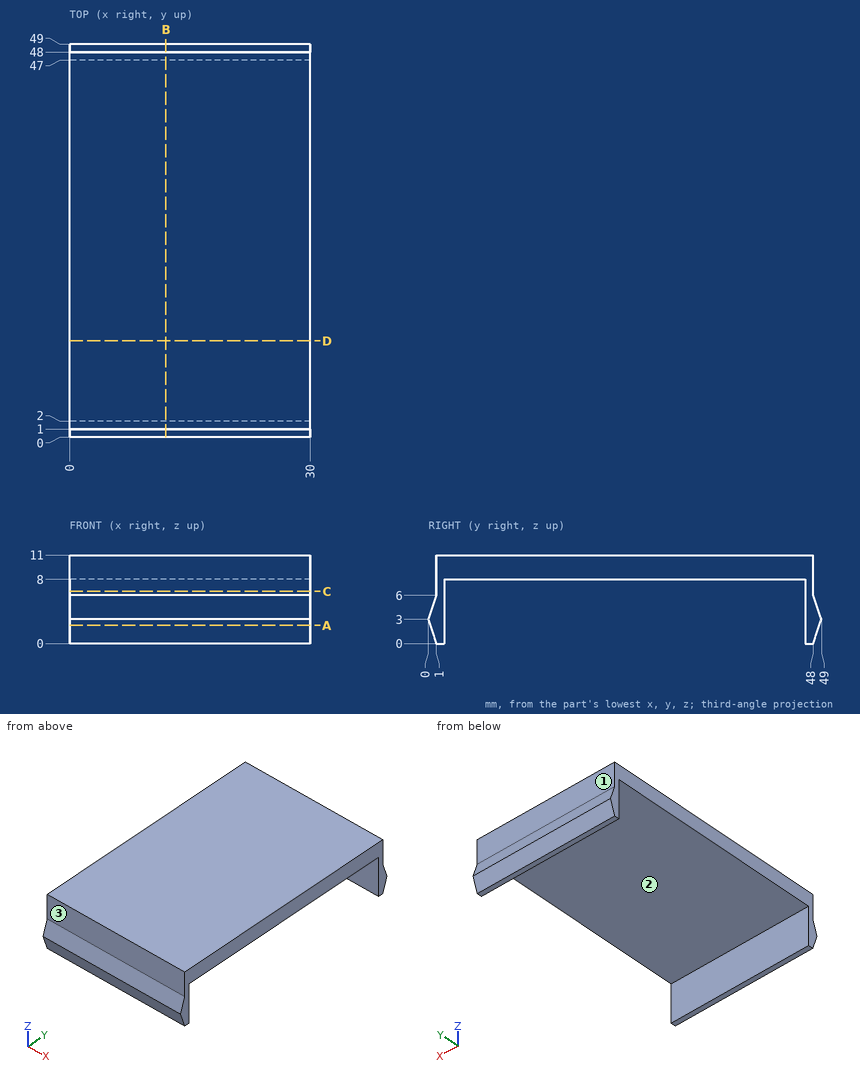
Design review of the part shown in the three views and the two pictorial views. Dimensions are in mm from the part's minimum x, y and z. A direction names the side the tool comes from. Round coordinates to 2 decimals unless told otherwise and drop trailing zeros. Loops run counter-clockwise (first coordinate to the right, second up) from the corner with the lowest first, then second, coordinate; pieces in that order, holes last. Notation, with made-up numbers: (-33.5, -20.75) -> (-17.5, -20.75) arc R18 ccw to (-17.5, 6.25) -> close; hole circle Ø1 at (42, -9). An arc over 180 degrees is marked (long way). Use one line per item in the form item = value. Start each with the question number.
Q1. Machinability: for the marked faces 1, 2 and 3, which of the approach directions +Z, -Z, +X, -X, +Y, -Y give a long, thin tool a straight path to every point of the face, cutting with its end or side? Answer none if there is none.
Q2. We need section B-B on x = 12. Give the boundary of the cut face in (y, z).
Q3. We need section C-C on z = 6.5. Give the boundary of the cut face in (x, y), then the cut area to 3 significant figures.
Q4. Wall thickness on line 1 along Y through (x, z) = (8.75, 7); line 2 along Y through (x, z) = (16, 4.5); line 3 along Z through (x, y) = (28, 32): over which ranges is each line inside the solid? List them lowest first. Write a range as [from, to].
Q5. For pin 1 Ø4 at (x, z) = (21.5, 9.5) entering from +Y; pin 2 Ø4 at (x, z) = (19, 9.5) entering from -Y; pin 3 Ø4 at (x, y) = (17.5, 38.5) entering from -Z, all flat-tipped, find the tip position at first contact; note any pin that passes through.
Q6. We need section D-D on y = 12. Give the boundary of the cut face in (x, z), then the cut area to 3 significant figures.
Q7. We need section A-A on z = 2.25. Give the boundary of the cut face in (x, y), then the cut area to 3 significant figures.
Calculated:
q1.face_1 = +Z, +X, -X, +Y
q1.face_2 = -Z, +X, -X
q1.face_3 = +Z, +X, -X, -Y
q2.outline = (0, 3) -> (1, 0) -> (2, 0) -> (2, 8) -> (47, 8) -> (47, 0) -> (48, 0) -> (49, 3) -> (48, 6) -> (48, 11) -> (1, 11) -> (1, 6) -> close
q3.outline = (0, 1) -> (30, 1) -> (30, 2) -> (0, 2) -> close; (0, 47) -> (30, 47) -> (30, 48) -> (0, 48) -> close
q3.area = 60.0 mm²
q4.line_1 = [1, 2], [47, 48]
q4.line_2 = [0.5, 2], [47, 48.5]
q4.line_3 = [8, 11]
q5.pin_1 = 48
q5.pin_2 = 1
q5.pin_3 = 8
q6.outline = (0, 8) -> (30, 8) -> (30, 11) -> (0, 11) -> close
q6.area = 90.0 mm²
q7.outline = (0, 0.25) -> (30, 0.25) -> (30, 2) -> (0, 2) -> close; (0, 47) -> (30, 47) -> (30, 48.75) -> (0, 48.75) -> close
q7.area = 105 mm²
